```python
from build123d import *

# Parameters (mm, degrees)
SKETCH1_W              = 50.8
SKETCH1_H              = 25.4
SKETCH1_W_2            = 47.498
SKETCH1_H_2            = 22.098
BOSS_EXTRUDE1_DEPTH    = 330
CUT_EXTRUDE5_REACH     = 27.4
SKETCH8_R              = 3.3
CUT_EXTRUDE6_DEPTH     = 26.4
F_00_CLEARANCE_HOLE1_D = 6.600000008


with BuildPart() as part:
    # Sketch1 → Boss-Extrude1 (new body)
    with BuildSketch(Plane.XY):
        Rectangle(SKETCH1_W, SKETCH1_H)
        Rectangle(SKETCH1_W_2, SKETCH1_H_2, mode=Mode.SUBTRACT)
    extrude(amount=BOSS_EXTRUDE1_DEPTH)

    # Sketch4 → Cut-Extrude5 (cut, up to next)
    with BuildSketch(Plane(origin=(0, 12.7, 0), x_dir=(1, 0, 0), z_dir=(0, 1, 0)), mode=Mode.PRIVATE) as cut_extrude5_sk1:
        with BuildLine():
            Line((-6, -270), (-6, -330))
            Line((-6, -330), (6, -330))
            Line((6, -330), (6, -270))
            ThreePointArc((6, -270), (0, -264), (-6, -270))
        make_face()
    cut_extrude5_tool1 = extrude(cut_extrude5_sk1.sketch, amount=-CUT_EXTRUDE5_REACH, mode=Mode.PRIVATE) & part.part
    add(cut_extrude5_tool1.solids().sort_by_distance((0, 12.7, 297.629949))[0], mode=Mode.SUBTRACT)

    # Sketch8 → Cut-Extrude6 (cut, through all)
    with BuildSketch(Plane(origin=(0, 12.7, 0), x_dir=(1, 0, 0), z_dir=(0, 1, 0))):
        with BuildLine():
            ThreePointArc((-9.427922061, -316.727922061), (-9.679119604, -315.465066735), (-10.394469683, -314.394469683))
            Line((-10.394469683, -314.394469683), (-15.061374439, -319.061374439))
            ThreePointArc((-15.061374439, -319.061374439), (-11.465066735, -319.776724519), (-9.427922061, -316.727922061))
        make_face()
        with BuildLine():
            Line((-15.061374439, -319.061374439), (-10.394469683, -314.394469683))
            ThreePointArc((-10.394469683, -314.394469683), (-15.061374439, -314.394469683), (-15.061374439, -319.061374439))
        make_face()
        with Locations((-12.727922061, -291.272077939)):
            Circle(SKETCH8_R)
        with Locations((12.727922061, -291.272077939)):
            Circle(SKETCH8_R)
        with Locations((12.727922061, -316.727922061)):
            Circle(SKETCH8_R)
    extrude(amount=-CUT_EXTRUDE6_DEPTH, mode=Mode.SUBTRACT)

    # #00 Clearance Hole1 (through all)
    with Locations(Plane(origin=(136.368987279, 20.7, -48.715791339), x_dir=(0.866025404, 0, -0.5), z_dir=(0, 1, 0))):
        with Locations((-156.901570158, 26.695380774), (-141.901570158, 8.695380774), (-171.901570158, 8.695380774)):
            Hole(F_00_CLEARANCE_HOLE1_D / 2)


solid = part.part
```
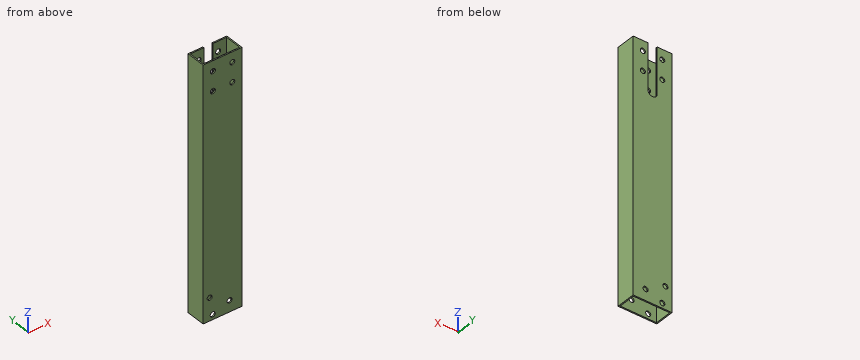
Geometry check sheet. Reference: the model listing, model coordinates, mm. Round coordinates to 2 decimals unless told otherwise and drop trailing zeros. Loops run counter-clockwise (first coordinate to the right, second up) from the corner with the lowest first, then second, coordinate; pieces in that order, holes last. Notation, with made-up numbers: (36, 62) - (75, 62) arc R4 ccw to (75, 66) - close; hole circle Ø11 at (-6, 2). An arc over 180 degrees is marked (long way). Write item = value, one per line. Start each with the question number.
1. Section check B-B on y = -2.25. Enter the section's corners in (x, z).
2. Section check C-C on z = 101.5. Enter the section's corners in (x, y).
3. Thickness scan on line 1 (Z direction, x = -12.5, y = 11.75); line 2 (Y direction, x = -18, z = 177); line 3 (X direction, y = 10.25, z = 271.5). Record the ranges inside material, lowest first.
4. Section check A-A on x = 0. Enter the section's corners in (y, z), then the cut area to 3 significant figures.
Working result:
q1.outline = (-25.4, 0) - (-23.75, 0) - (-23.75, 330) - (-25.4, 330) - close; (23.75, 0) - (25.4, 0) - (25.4, 330) - (23.75, 330) - close
q2.outline = (-25.4, -12.7) - (25.4, -12.7) - (25.4, 12.7) - (-25.4, 12.7) - close; hole (-23.75, -11.05) - (23.75, -11.05) - (23.75, 11.05) - (-23.75, 11.05) - close
q3.line_1 = 0 to 3.34, 9.9 to 287.98, 294.56 to 313.44, 320.02 to 330
q3.line_2 = -12.7 to -11.05, 11.05 to 12.7
q3.line_3 = -25.4 to -23.75, 23.75 to 25.4
q4.outline = (-12.7, 0) - (-11.05, 0) - (-11.05, 330) - (-12.7, 330) - close; (11.05, 0) - (12.7, 0) - (12.7, 264) - (11.05, 264) - close
q4.area = 981 mm^2
